For this review, use the dimensioned drawing (mm, ordinates from the lowest corner) and the shaded views. A direction names the side the tool comes from. Give positions to 0.01 mm unless a question says otherwise; leave off trailing zeros. Write each loop counter-clockwise with the first axis right and the second up, starting at its lowest first coordinate (ties: lowest second). Pieces come first, ordered by that corner, then holes.
1) Machinability: for the marked faces 1 and 2, which of the approach directions +Z, -Z, +X, -X, +Y, -Y give a long, thin tool a straight path to every point of the face, cutting with its end or side? Answer none if there is none.
2) For P1, Ø6, axis at x = 35, z = 5, coming from the +Y side; P2, Ø12, axis at x = 52, z = 10, coming from the -Y side; P3, Ø3.5, axis at x = 35, z = 65, coming from the +Y side; P4, Ø4, axis at x = 49, y = 45.5, coming from the -Z side, all flat-tipped, find the tip position at first contact; note any pin that passes through.
3) We need section D-D on x = 56. Give the boundary of the cut face in (y, z).
4) We need section C-C on z = 48.5. Give the boundary of the cut face in (x, y).
5) We need section A-A on x = 35. Give the boundary of the cut face in (y, z), and give its area (3 significant figures).
6) We need section B-B on z = 5. Give the boundary of the cut face in (x, y).
7) Wall thickness on line 1 along Z through (x, y) = (35, 53.75); line 2 along Y through (x, z) = (27, 19); line 3 along X through (y, z) = (54, 5): over which ranges is each line inside the solid? List them lowest first.
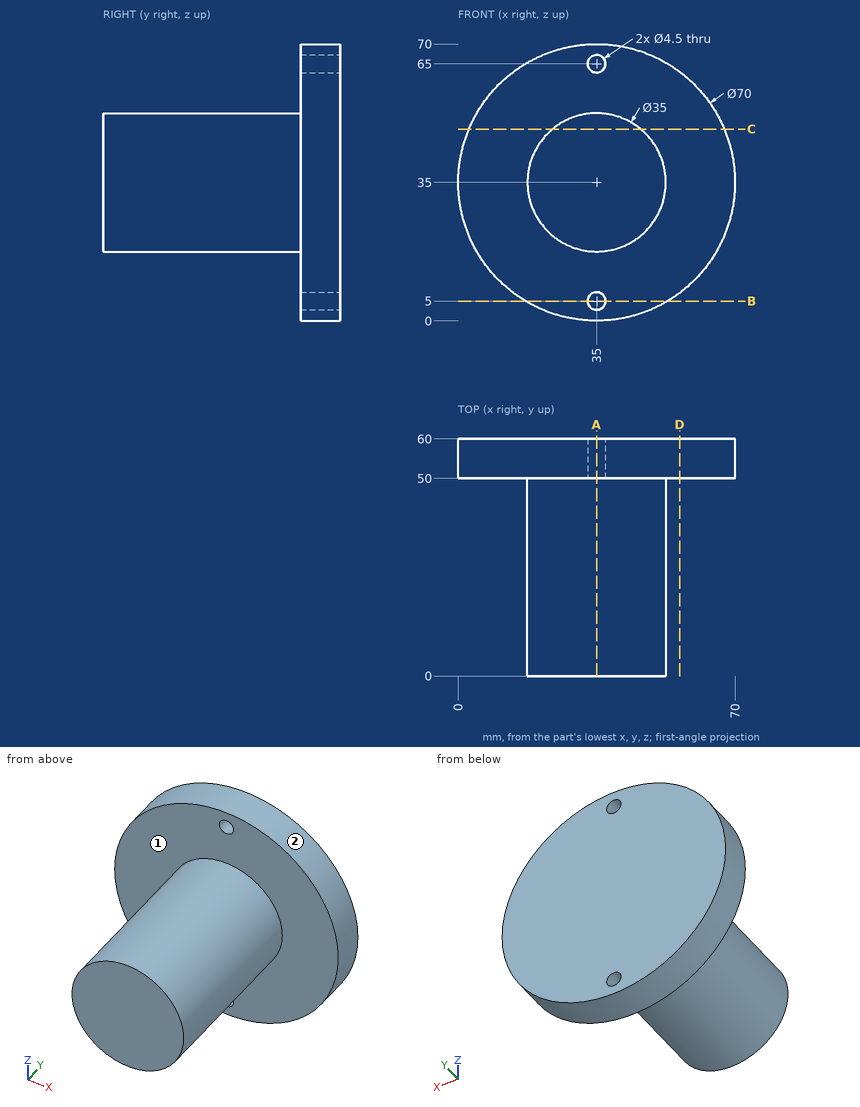
Results list:
1. face 1: -Y
1. face 2: +Y, -Y
2. P1: stops at y = 60
2. P2: stops at y = 50
2. P3: passes through
2. P4: stops at z = 22.26
3. outline: (50, 7) - (60, 7) - (60, 63) - (50, 63) - close
4. outline: (2.71, 50) - (23.86, 50) - (23.86, 0) - (46.14, 0) - (46.14, 50) - (67.29, 50) - (67.29, 60) - (2.71, 60) - close
5. outline: (0, 17.5) - (50, 17.5) - (50, 7.25) - (60, 7.25) - (60, 62.75) - (50, 62.75) - (50, 52.5) - (0, 52.5) - close; (50, 0) - (60, 0) - (60, 2.75) - (50, 2.75) - close; (50, 67.25) - (60, 67.25) - (60, 70) - (50, 70) - close
5. area: 2,360 mm2
6. outline: (16.97, 50) - (32.75, 50) - (32.75, 60) - (16.97, 60) - close; (37.25, 50) - (53.03, 50) - (53.03, 60) - (37.25, 60) - close
7. line 1: z = 0 to 2.75, 7.25 to 62.75, 67.25 to 70
7. line 2: y = 50 to 60
7. line 3: x = 16.97 to 32.75, 37.25 to 53.03
